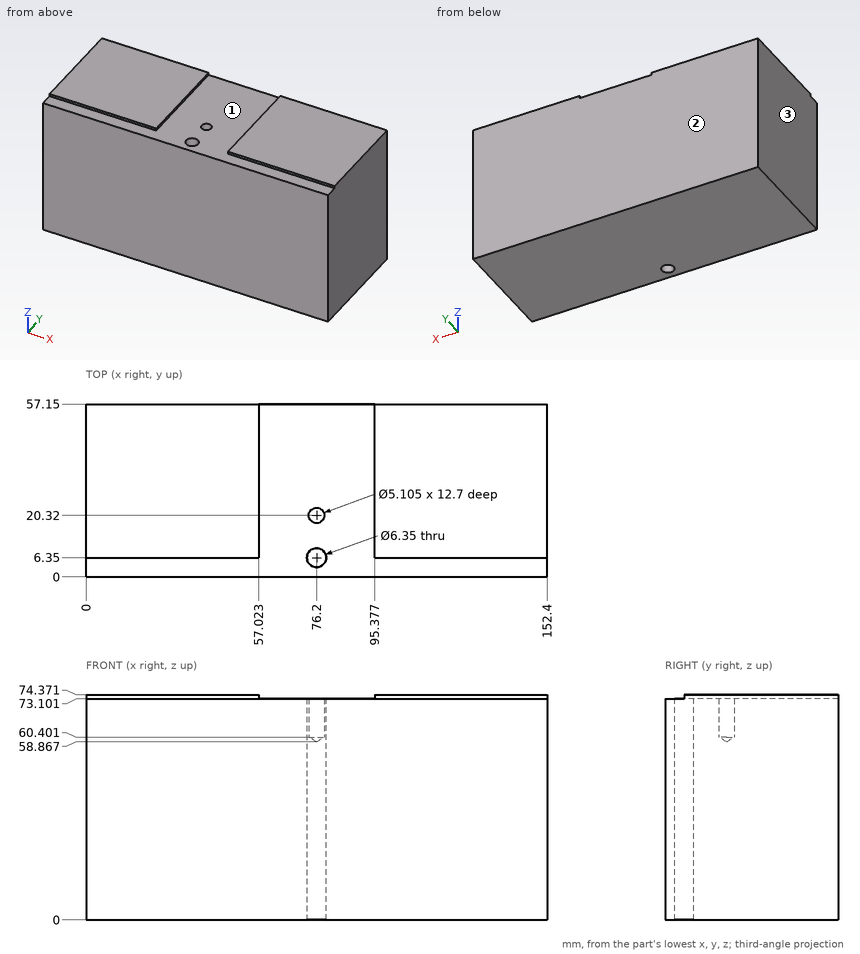
Could you check a few things on this drawing? It's one solid part, dimensions in mm from its lowest x, y, z. Give positions to 0.01 mm unless a question says otherwise; leave off trailing zeros. One line per question, with ' | ' between items. Start each with the question number.
Item 1: I need wall thicknesses on probe 1 along X at (y, z) = (6.35, 19) (1 decimal); probe 2 along X at (y, z) = (20.32, 69); probe 3 along Y at (x, z) = (76, 27). Which ranges of each line are inside material? Lowest first, please. Write a range as [from, to].
Item 2: I'm going to push flat-ended pins straight in: pin 1 Ø4 at (x, y) = (76.2, 20.32) entering from -Z; pin 2 Ø10 at (x, y) = (76.2, 6.35) entering from +Z. Where does each tip first touch, or does it pass through?
Item 3: Thinking about a two-plate mould opening in X: for the marked faces 1, 2 and 3, which applies, pulls with the +X half, pulls with the -X half, needs draft (parallel to the pull), parting line crosses it, or undercut?
Verdict:
1) probe 1: [0, 73], [79.4, 152.4] | probe 2: [0, 73.65], [78.75, 152.4] | probe 3: [0, 3.18], [9.52, 57.15]
2) pin 1: z = 0 | pin 2: z = 73.1
3) face 1: undercut | face 2: needs draft | face 3: pulls with the -X half
